Autodesk Inventor part; units mm, degrees
ref_plane "YZ Plane" through (0, 0, 0) normal (1, 0, 0) x (0, 1, 0)
ref_plane "XZ Plane" through (0, 0, 0) normal (0, 1, 0) x (-1, 0, 0)
ref_plane "XY Plane" through (0, 0, 0) normal (0, 0, 1) x (1, 0, 0)
sketch "Sketch1" plane through (0, 0, 0) normal (1, 0, 0) x (0, 1, 0)
  line L0 (-7.5, -7.5) -> (7.5, -7.5)
  line L1 (7.5, -7.5) -> (7.5, 7.5)
  line L2 (7.5, 7.5) -> (-7.5, 7.5)
  line L3 (-7.5, 7.5) -> (-7.5, -7.5)
  line L4 (-7.5, -7.5) -> (7.5, 7.5) construction
  line L5 (7.5, -7.5) -> (-7.5, 7.5) construction
  line L6 (7.5, 1.5) -> (4.5, 1.5)
  line L7 (4.5, 1.5) -> (4.5, -1.5)
  line L8 (4.5, -1.5) -> (7.5, -1.5)
  line L9 (7.5, -1.5) -> (7.5, 1.5)
  line L10 (1.5, 7.5) -> (-1.5, 7.5)
  line L11 (-1.5, 7.5) -> (-1.5, 4.5)
  line L12 (-1.5, 4.5) -> (1.5, 4.5)
  line L13 (1.5, 4.5) -> (1.5, 7.5)
  line L14 (-7.5, 1.5) -> (-4.5, 1.5)
  line L15 (-4.5, 1.5) -> (-4.5, -1.5)
  line L16 (-4.5, -1.5) -> (-7.5, -1.5)
  line L17 (-7.5, -1.5) -> (-7.5, 1.5)
  line L18 (-1.5, -7.5) -> (1.5, -7.5)
  line L19 (1.5, -7.5) -> (1.5, -4.5)
  line L20 (1.5, -4.5) -> (-1.5, -4.5)
  line L21 (-1.5, -4.5) -> (-1.5, -7.5)
  point P0 (0, 0)
  dimension "d0" = 15
  dimension "d1" = 3
  dimension "d2" = 3
  dimension "d3" = 1.5
  dimension "d4" = 1.5
extrude "Extrusion1" add sketch "Sketch1" along normal blind 500 contours L3 L16 L15 L14 L2 L11 L12 L13 L1 L6 L7 L8 L0 L19 L20 L21
properties part number "Beam_360mm" material "Aluminum 6061"
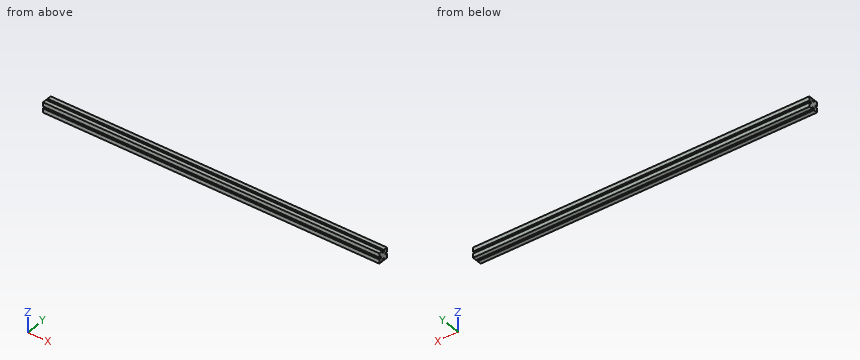
The model under review builds one solid part; all positions refer to its coordinate system, in mm. Give positions to 0.01 mm unless a question says otherwise; leave off trailing zeros. Order: outer loops, then holes, each group sorted by start corner. A loop starts at its lowest first (then second) coordinate and runs counter-clockwise, first axis right, second up. Notation, with made-up numbers: M 61.25,26 L 97.25,26 A23 ccw 97.25,40 Z; hole C 49.5,-37 d4. An arc over 180 degrees is marked long. Answer in a Markdown table with one row per item. Add a question column.
1. For pin 1 Ø1.5 at (x, z) = (182, 0.5) entering from -Y; pin 2 Ø1.5 at (x, y) = (294, 0.5) entering from -Z; pin 3 Ø0.9 at (x, z) = (327.5, 0.5) entering from +Y, all flat-tipped, find the tip position at first contact; note any pin that passes through.
2. To check wall thickness, follow line 1 along Z through (x, y) = (391, -4.75); line 2 along Y through (x, z) = (347, 1.25). State the ranges of each line that lie inside material, in increasing order.
3. Add section A-A on x = 327. State the section outline as (y, z) points, plus the area to 3 significant figures.
The answers:
| question | item | result |
|---|---|---|
| 1 | pin 1 | y = -4.5 |
| 1 | pin 2 | z = -4.5 |
| 1 | pin 3 | y = 4.5 |
| 2 | line 1 | -7.5 to -1.5, 1.5 to 7.5 |
| 2 | line 2 | -4.5 to 4.5 |
| 3 | outline | M -7.5,-7.5 L -1.5,-7.5 L -1.5,-4.5 L 1.5,-4.5 L 1.5,-7.5 L 7.5,-7.5 L 7.5,-1.5 L 4.5,-1.5 L 4.5,1.5 L 7.5,1.5 L 7.5,7.5 L 1.5,7.5 L 1.5,4.5 L -1.5,4.5 L -1.5,7.5 L -7.5,7.5 L -7.5,1.5 L -4.5,1.5 L -4.5,-1.5 L -7.5,-1.5 Z |
| 3 | area | 189 mm2 |
